from build123d import *

# Parameters (mm, degrees)
F0_W          = 20
F0_H          = 20.6382983719
F1_DEPTH      = 10
F2_R          = 2
F3_DEPTH      = 3
F4_R          = 2
F5_DEPTH      = 3
F6_R          = 2
F7_DEPTH      = 3
F8_R          = 2
F9_DEPTH      = 3
F10_R         = 2
F11_DEPTH     = 3
F12_R         = 2
F13_DEPTH     = 3
F14_T1_DEPTH  = 16
F14_T3_DEPTH  = 16
F14_T5_DEPTH  = 16.6382983719
F14_S9_W      = 2
F14_S9_H      = 2
F14_T10_DEPTH = 2
F14_S15_W     = 2
F14_S15_H     = 2
F14_T16_DEPTH = 2
F14_S21_W     = 2
F14_S21_H     = 2
F14_T22_DEPTH = 2
F14_S27_W     = 2
F14_S27_H     = 2
F14_T28_DEPTH = 2
F14_S33_W     = 2
F14_S33_H     = 2
F14_T34_DEPTH = 2
F14_S39_W     = 2
F14_S39_H     = 2
F14_T40_DEPTH = 2
F14_S45_W     = 2
F14_S45_H     = 2
F14_T46_DEPTH = 2
F14_S51_W     = 2
F14_S51_H     = 2
F14_T52_DEPTH = 2


# Not quite as in the source:
# - a fillet or chamfer that OpenCascade refuses, or shapes differently, is made with other operations: its cross-section is extruded or revolved along the edge and cut away or added


with BuildPart() as f1:
    # F0 (on Top) → F1 (new body, symmetric)
    with BuildSketch(Plane.XY):
        with Locations((0.4536276683, -0.0907257199)):
            Rectangle(F0_W, F0_H)
    extrude(amount=F1_DEPTH, both=True)

    # F2 (on face) → F3 (cut)
    with BuildSketch(Plane.XY.offset(10)):
        Circle(F2_R)
    extrude(amount=-F3_DEPTH, mode=Mode.SUBTRACT)

    # F4 (on face) → F5 (cut)
    with BuildSketch(Plane(origin=(0, 0, -10), x_dir=(1, 0, 0), z_dir=(0, 0, -1))):
        with Locations((-5.7126359213, 5.4597818985)):
            Circle(F4_R)
        with Locations((0, 5.5342745036)):
            Circle(F4_R)
        with Locations((6.2873640787, 5.4597818985)):
            Circle(F4_R)
        with Locations((-5.3870321827, -4.9442961443)):
            Circle(F4_R)
        with Locations((0, -4.9442961443)):
            Circle(F4_R)
        with Locations((5.8821875854, -4.9210169871)):
            Circle(F4_R)
    extrude(amount=-F5_DEPTH, mode=Mode.SUBTRACT)

    # F6 (on face) → F7 (cut)
    with BuildSketch(Plane(origin=(-9.5463723317, 0, 0), x_dir=(0, -1, 0), z_dir=(-1, 0, 0))):
        with Locations((0.0200922749, 5.65356597)):
            Circle(F6_R)
        with Locations((0, -5.5342745036)):
            Circle(F6_R)
    extrude(amount=-F7_DEPTH, mode=Mode.SUBTRACT)

    # F8 (on face) → F9 (cut)
    with BuildSketch(Plane.YZ.offset(10.4536276683)):
        Circle(F8_R)
        with Locations((-5.3528235294, 5.5342745036)):
            Circle(F8_R)
        with Locations((5.3528235294, 5.5342745036)):
            Circle(F8_R)
        with Locations((-5.3528235294, -5.5342745036)):
            Circle(F8_R)
        with Locations((5.3528235294, -5.5342745036)):
            Circle(F8_R)
    extrude(amount=-F9_DEPTH, mode=Mode.SUBTRACT)

    # F10 (on face) → F11 (cut)
    with BuildSketch(Plane(origin=(0, 10.228423466, 0), x_dir=(-1, 0, 0), z_dir=(0, 1, 0))):
        with Locations((0.0112662294, -0.0190863853)):
            Circle(F10_R)
        with Locations((4.8084682785, -4.8084678128)):
            Circle(F10_R)
        with Locations((-5.254099916, 4.9555348842)):
            Circle(F10_R)
    extrude(amount=-F11_DEPTH, mode=Mode.SUBTRACT)

    # F12 (on face) → F13 (cut)
    with BuildSketch(Plane.XZ.offset(10.4098749059)):
        with Locations((5.1735501704, 5.0105248782)):
            Circle(F12_R)
        with Locations((-5.1735501704, 5.0105248782)):
            Circle(F12_R)
        with Locations((-5.1735501704, -5.0105248782)):
            Circle(F12_R)
        with Locations((5.1735501704, -5.0105248782)):
            Circle(F12_R)
    extrude(amount=-F13_DEPTH, mode=Mode.SUBTRACT)

    # F14: fillet of radius 2 on 12 edges, made by hand

    # F14_s2 → F14_t1 (cut)
    with BuildSketch(Plane.XY.offset(-8)):
        with BuildLine():
            ThreePointArc((10.4536276683, -8.4098749059), (9.8678412307, -9.8240884682), (8.4536276683, -10.4098749059))
            Line((8.4536276683, -10.4098749059), (10.4536276683, -10.4098749059))
            Line((10.4536276683, -10.4098749059), (10.4536276683, -8.4098749059))
        make_face()
        with BuildLine():
            ThreePointArc((-9.5463723317, -8.4098749059), (-8.9605858941, -9.8240884682), (-7.5463723317, -10.4098749059))
            Line((-7.5463723317, -10.4098749059), (-9.5463723317, -10.4098749059))
            Line((-9.5463723317, -10.4098749059), (-9.5463723317, -8.4098749059))
        make_face()
        with BuildLine():
            ThreePointArc((-7.5463723317, 10.228423466), (-8.9605858941, 9.6426370284), (-9.5463723317, 8.228423466))
            Line((-9.5463723317, 8.228423466), (-9.5463723317, 10.228423466))
            Line((-9.5463723317, 10.228423466), (-7.5463723317, 10.228423466))
        make_face()
        with BuildLine():
            ThreePointArc((8.4536276683, 10.228423466), (9.8678412307, 9.6426370284), (10.4536276683, 8.228423466))
            Line((10.4536276683, 8.228423466), (10.4536276683, 10.228423466))
            Line((10.4536276683, 10.228423466), (8.4536276683, 10.228423466))
        make_face()
    extrude(amount=F14_T1_DEPTH, mode=Mode.SUBTRACT)

    # F14_s4 → F14_t3 (cut)
    with BuildSketch(Plane.YZ.offset(-7.5463723317)):
        with BuildLine():
            ThreePointArc((-8.4098749059, 10), (-9.8240884682, 9.4142135624), (-10.4098749059, 8))
            Line((-10.4098749059, 8), (-10.4098749059, 10))
            Line((-10.4098749059, 10), (-8.4098749059, 10))
        make_face()
        with BuildLine():
            ThreePointArc((-8.4098749059, -10), (-9.8240884682, -9.4142135624), (-10.4098749059, -8))
            Line((-10.4098749059, -8), (-10.4098749059, -10))
            Line((-10.4098749059, -10), (-8.4098749059, -10))
        make_face()
        with BuildLine():
            ThreePointArc((10.228423466, -8), (9.6426370284, -9.4142135624), (8.228423466, -10))
            Line((8.228423466, -10), (10.228423466, -10))
            Line((10.228423466, -10), (10.228423466, -8))
        make_face()
        with BuildLine():
            ThreePointArc((10.228423466, 8), (9.6426370284, 9.4142135624), (8.228423466, 10))
            Line((8.228423466, 10), (10.228423466, 10))
            Line((10.228423466, 10), (10.228423466, 8))
        make_face()
    extrude(amount=F14_T3_DEPTH, mode=Mode.SUBTRACT)

    # F14_s6 → F14_t5 (cut)
    with BuildSketch(Plane.XZ.offset(-8.228423466)):
        with BuildLine():
            ThreePointArc((-9.5463723317, 8), (-8.9605858941, 9.4142135624), (-7.5463723317, 10))
            Line((-7.5463723317, 10), (-9.5463723317, 10))
            Line((-9.5463723317, 10), (-9.5463723317, 8))
        make_face()
        with BuildLine():
            ThreePointArc((-7.5463723317, -10), (-8.9605858941, -9.4142135624), (-9.5463723317, -8))
            Line((-9.5463723317, -8), (-9.5463723317, -10))
            Line((-9.5463723317, -10), (-7.5463723317, -10))
        make_face()
        with BuildLine():
            ThreePointArc((8.4536276683, -10), (9.8678412307, -9.4142135624), (10.4536276683, -8))
            Line((10.4536276683, -8), (10.4536276683, -10))
            Line((10.4536276683, -10), (8.4536276683, -10))
        make_face()
        with BuildLine():
            ThreePointArc((10.4536276683, 8), (9.8678412307, 9.4142135624), (8.4536276683, 10))
            Line((8.4536276683, 10), (10.4536276683, 10))
            Line((10.4536276683, 10), (10.4536276683, 8))
        make_face()
    extrude(amount=F14_T5_DEPTH, mode=Mode.SUBTRACT)


with BuildPart() as f14_tool8:
    # F14_s9 → F14_t10 (new body)
    with BuildSketch(Plane.XZ.offset(8.4098749059)):
        with Locations((9.4536276683, 9)):
            Rectangle(F14_S9_W, F14_S9_H)
    extrude(amount=F14_T10_DEPTH)

    # F14_s11 → F14_t12 (revolve, cut)
    with BuildSketch(Plane(origin=(8.4536276683, -8.4098749059, 8), x_dir=(-0.7071067812, 0, -0.7071067812), z_dir=(-0.7071067812, 0, 0.7071067812))):
        with BuildLine():
            ThreePointArc((0, -2), (2, 0), (0, 2))
            Line((0, 2), (0, -2))
        make_face()
    revolve(axis=Axis((8.4536276683, -8.4098749059, 8), (0, -1, 0)), mode=Mode.SUBTRACT)


with BuildPart() as f1_1:
    add(f1.part)

    # F14_t7: cut F14_tool8
    add(f14_tool8.part, mode=Mode.SUBTRACT)


with BuildPart() as f14_tool14:
    # F14_s15 → F14_t16 (new body)
    with BuildSketch(Plane.XZ.offset(8.4098749059)):
        with Locations((9.4536276683, -9)):
            Rectangle(F14_S15_W, F14_S15_H)
    extrude(amount=F14_T16_DEPTH)

    # F14_s17 → F14_t18 (revolve, cut)
    with BuildSketch(Plane(origin=(8.4536276683, -8.4098749059, -8), x_dir=(-0.7071067812, 0, 0.7071067812), z_dir=(0.7071067812, 0, 0.7071067812))):
        with BuildLine():
            ThreePointArc((0, -2), (2, 0), (0, 2))
            Line((0, 2), (0, -2))
        make_face()
    revolve(axis=Axis((8.4536276683, -8.4098749059, -8), (0, -1, 0)), mode=Mode.SUBTRACT)


with BuildPart() as f1_2:
    add(f1_1.part)

    # F14_t13: cut F14_tool14
    add(f14_tool14.part, mode=Mode.SUBTRACT)


with BuildPart() as f14_tool20:
    # F14_s21 → F14_t22 (new body)
    with BuildSketch(Plane.XZ.offset(8.4098749059)):
        with Locations((-8.5463723317, 9)):
            Rectangle(F14_S21_W, F14_S21_H)
    extrude(amount=F14_T22_DEPTH)

    # F14_s23 → F14_t24 (revolve, cut)
    with BuildSketch(Plane(origin=(-7.5463723317, -8.4098749059, 8), x_dir=(0.7071067812, 0, -0.7071067812), z_dir=(-0.7071067812, 0, -0.7071067812))):
        with BuildLine():
            ThreePointArc((0, -2), (2, 0), (0, 2))
            Line((0, 2), (0, -2))
        make_face()
    revolve(axis=Axis((-7.5463723317, -8.4098749059, 8), (0, -1, 0)), mode=Mode.SUBTRACT)


with BuildPart() as f1_3:
    add(f1_2.part)

    # F14_t19: cut F14_tool20
    add(f14_tool20.part, mode=Mode.SUBTRACT)


with BuildPart() as f14_tool26:
    # F14_s27 → F14_t28 (new body)
    with BuildSketch(Plane.XZ.offset(8.4098749059)):
        with Locations((-8.5463723317, -9)):
            Rectangle(F14_S27_W, F14_S27_H)
    extrude(amount=F14_T28_DEPTH)

    # F14_s29 → F14_t30 (revolve, cut)
    with BuildSketch(Plane(origin=(-7.5463723317, -8.4098749059, -8), x_dir=(0.7071067812, 0, 0.7071067812), z_dir=(0.7071067812, 0, -0.7071067812))):
        with BuildLine():
            ThreePointArc((0, -2), (2, 0), (0, 2))
            Line((0, 2), (0, -2))
        make_face()
    revolve(axis=Axis((-7.5463723317, -8.4098749059, -8), (0, -1, 0)), mode=Mode.SUBTRACT)


with BuildPart() as f1_4:
    add(f1_3.part)

    # F14_t25: cut F14_tool26
    add(f14_tool26.part, mode=Mode.SUBTRACT)


with BuildPart() as f14_tool32:
    # F14_s33 → F14_t34 (new body)
    with BuildSketch(Plane.XZ.offset(-8.228423466)):
        with Locations((-8.5463723317, 9)):
            Rectangle(F14_S33_W, F14_S33_H)
    extrude(amount=-F14_T34_DEPTH)

    # F14_s35 → F14_t36 (revolve, cut)
    with BuildSketch(Plane(origin=(-7.5463723317, 8.228423466, 8), x_dir=(0.7071067812, 0, -0.7071067812), z_dir=(0.7071067812, 0, 0.7071067812))):
        with BuildLine():
            ThreePointArc((0, -2), (2, 0), (0, 2))
            Line((0, 2), (0, -2))
        make_face()
    revolve(axis=Axis((-7.5463723317, 8.228423466, 8), (0, 1, 0)), mode=Mode.SUBTRACT)


with BuildPart() as f1_5:
    add(f1_4.part)

    # F14_t31: cut F14_tool32
    add(f14_tool32.part, mode=Mode.SUBTRACT)


with BuildPart() as f14_tool38:
    # F14_s39 → F14_t40 (new body)
    with BuildSketch(Plane.XZ.offset(-8.228423466)):
        with Locations((-8.5463723317, -9)):
            Rectangle(F14_S39_W, F14_S39_H)
    extrude(amount=-F14_T40_DEPTH)

    # F14_s41 → F14_t42 (revolve, cut)
    with BuildSketch(Plane(origin=(-7.5463723317, 8.228423466, -8), x_dir=(0.7071067812, 0, 0.7071067812), z_dir=(-0.7071067812, 0, 0.7071067812))):
        with BuildLine():
            ThreePointArc((0, -2), (2, 0), (0, 2))
            Line((0, 2), (0, -2))
        make_face()
    revolve(axis=Axis((-7.5463723317, 8.228423466, -8), (0, 1, 0)), mode=Mode.SUBTRACT)


with BuildPart() as f1_6:
    add(f1_5.part)

    # F14_t37: cut F14_tool38
    add(f14_tool38.part, mode=Mode.SUBTRACT)


with BuildPart() as f14_tool44:
    # F14_s45 → F14_t46 (new body)
    with BuildSketch(Plane.XZ.offset(-8.228423466)):
        with Locations((9.4536276683, -9)):
            Rectangle(F14_S45_W, F14_S45_H)
    extrude(amount=-F14_T46_DEPTH)

    # F14_s47 → F14_t48 (revolve, cut)
    with BuildSketch(Plane(origin=(8.4536276683, 8.228423466, -8), x_dir=(-0.7071067812, 0, 0.7071067812), z_dir=(-0.7071067812, 0, -0.7071067812))):
        with BuildLine():
            ThreePointArc((0, -2), (2, 0), (0, 2))
            Line((0, 2), (0, -2))
        make_face()
    revolve(axis=Axis((8.4536276683, 8.228423466, -8), (0, 1, 0)), mode=Mode.SUBTRACT)


with BuildPart() as f1_7:
    add(f1_6.part)

    # F14_t43: cut F14_tool44
    add(f14_tool44.part, mode=Mode.SUBTRACT)


with BuildPart() as f14_tool50:
    # F14_s51 → F14_t52 (new body)
    with BuildSketch(Plane.XZ.offset(-8.228423466)):
        with Locations((9.4536276683, 9)):
            Rectangle(F14_S51_W, F14_S51_H)
    extrude(amount=-F14_T52_DEPTH)

    # F14_s53 → F14_t54 (revolve, cut)
    with BuildSketch(Plane(origin=(8.4536276683, 8.228423466, 8), x_dir=(-0.7071067812, 0, -0.7071067812), z_dir=(0.7071067812, 0, -0.7071067812))):
        with BuildLine():
            ThreePointArc((0, -2), (2, 0), (0, 2))
            Line((0, 2), (0, -2))
        make_face()
    revolve(axis=Axis((8.4536276683, 8.228423466, 8), (0, 1, 0)), mode=Mode.SUBTRACT)


with BuildPart() as f1_8:
    add(f1_7.part)

    # F14_t49: cut F14_tool50
    add(f14_tool50.part, mode=Mode.SUBTRACT)


solid = f1_8.part
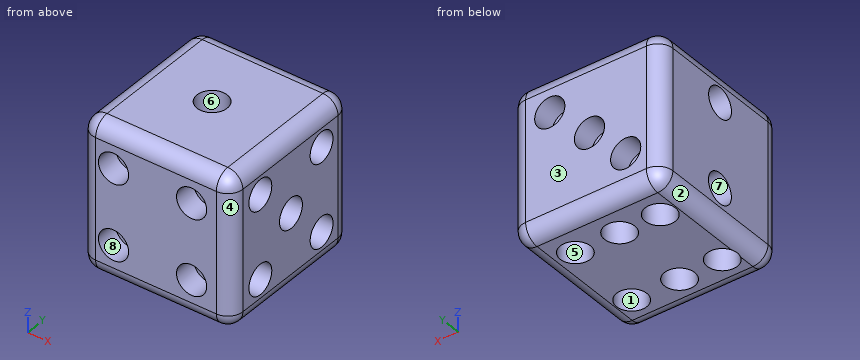
Input: part model. Units: mm. Frame: model coordinates. Face numbers are marked on the shaded views. A direction names the side the tool comes from. Round coordinates to 2 decimals unless told otherwise and drop trailing zeros. Order: outer loops, then holes, each group sorted by start corner. A loop starts at its lowest first (then second) coordinate and runs counter-clockwise, first axis right, second up.
1. Material intervals for line 1 (X direction, y = -8.5, z = 5); line 2 (Y direction, x = 0, z = 8.1); line 3 (Y direction, x = -6.5, z = -9), sorted ascending.
The answers:
line 1: x = -9.54 to -7.17, -3.17 to 3.17, 7.17 to 10.45
line 2: y = -10.41 to -2, 2 to 10.23
line 3: y = -10.14 to -7.3, -3.62 to 3.28, 6.61 to 9.96
2. Cut plane D-D, the plane y = 0. Output: boundary loops of the cut face in (x, z).
The answers:
outline: (-9.55, -8) arc R2 ccw to (-7.55, -10) - (8.45, -10) arc R2 ccw to (10.45, -8) - (10.45, -2) - (7.45, -2) - (7.45, 2) - (10.45, 2) - (10.45, 8) arc R2 ccw to (8.45, 10) - (2, 10) - (2, 7) - (-2, 7) - (-2, 10) - (-7.55, 10) arc R2 ccw to (-9.55, 8) - (-9.55, 7.65) - (-6.55, 7.65) - (-6.55, 3.65) - (-9.55, 3.65) - (-9.55, -3.53) - (-6.55, -3.53) - (-6.55, -7.53) - (-9.55, -7.53) - close
3. Set-up query: the marked faces 5, 6, 7 and 8. Return all of +Z, -Z, +X, -X, +Y, -Y with unobstructed straight access to the full face (end or side cutting, diameter ignored); none if empty.
The answers:
face 5: -Z
face 6: +Z
face 7: -X
face 8: -Y
4. Pin query (flat end, axial travel): P1, Ø1.2, axis at x = -5.5, z = -4.5, coming from the -Y side; P2, Ø2.5, axis at x = 6.29, y = -5.46, coming from the -Z side; P3, Ø2.5, axis at x = 5.17, z = 5.01, coming from the +Y side. Return the tip coordinate at first contact, or that it passes through.
The answers:
P1: stops at y = -7.41
P2: stops at z = -7
P3: stops at y = 7.23
5. Mould query, pull axis Y, two halves, no side actions, for the marked faces 1, 2, 3 and 4. Classes: released by +Y, released by -Y, zero draft, split by the parting line, or undercut.
The answers:
face 1: undercut
face 2: zero draft
face 3: released by +Y
face 4: released by -Y
6. Cut plane A-A, the plane y = 5.75. Output: boundary loops of the cut face in (x, z), then the cut area to 3 significant figures.
The answers:
outline: (-9.55, -8) arc R2 ccw to (-7.55, -10) - (-7.22, -10) - (-7.22, -7) - (-3.56, -7) - (-3.56, -10) - (-1.83, -10) - (-1.83, -7) - (1.83, -7) - (1.83, -10) - (4.06, -10) - (4.06, -7) - (7.45, -7) - (7.45, -3.57) - (10.45, -3.57) - (10.45, 3.57) - (7.45, 3.57) - (7.45, 7.49) - (10.45, 7.49) - (10.45, 8) arc R2 ccw to (8.45, 10) - (-7.55, 10) arc R2 ccw to (-9.55, 8) - close; (7.7, -10) - (8.45, -10) arc R2 ccw to (10.45, -8) - (10.45, -7.49) - (7.7, -7.49) - close
area: 340 mm2
7. Cut plane C-C, the plane x = 0. Output: boundary loops of the cut face in (y, z), then the cut area to 3 significant figures.
The answers:
outline: (-10.41, -8) arc R2 ccw to (-8.41, -10) - (-7.53, -10) - (-7.53, -7) - (-3.53, -7) - (-3.53, -10) - (2.94, -10) - (2.94, -7) - (6.94, -7) - (6.94, -10) - (8.23, -10) arc R2 ccw to (10.23, -8) - (10.23, -2.02) - (7.23, -2.02) - (7.23, 1.98) - (10.23, 1.98) - (10.23, 8) arc R2 ccw to (8.23, 10) - (2, 10) - (2, 7) - (-2, 7) - (-2, 10) - (-8.41, 10) arc R2 ccw to (-10.41, 8) - close
area: 361 mm2
